from build123d import *

# Parameters (mm, degrees)
SKETCH1_R           = 1.077630735
BOSS_EXTRUDE1_DEPTH = 8.001
SKETCH4_R           = 2.032
CUT_EXTRUDE1_DEPTH  = 50.8
SKETCH5_R           = 3.048
CUT_EXTRUDE2_DEPTH  = 4.572
CUT_EXTRUDE4_DEPTH  = 34.909144773
FILLET2_R           = 5.08
FILLET3_R           = 1.6002
CHAMFER1_SIZE       = 0.508


with BuildPart() as part:
    # Sketch1 → Boss-Extrude1 (new body)
    with BuildSketch(Plane(origin=(0, 0, 0), x_dir=(1, 0, 0), z_dir=(0, 1, 0))):
        with BuildLine():
            Line((-0.609859659, 0), (0, 0))
            Line((0, 0), (4.662509606, 0))
            Line((4.662509606, 0), (4.662509606, -27.178))
            Line((4.662509606, -27.178), (8.472509606, -27.178))
            Line((8.472509606, -27.178), (8.472509606, 7.747))
            Line((8.472509606, 7.747), (4.535509606, 7.747))
            Line((4.535509606, 7.747), (-1.371859637, 1.839630756))
            ThreePointArc((-1.371859637, 1.839630756), (-0.197468217, 2.073231708), (0.467771075, 1.077630735))
            ThreePointArc((0.467771075, 1.077630735), (0.152140341, 0.315630735), (-0.609859659, 0))
        make_face()
        with Locations((-0.609859659, 1.077630735)):
            Circle(SKETCH1_R)
    boss_extrude1 = extrude(amount=BOSS_EXTRUDE1_DEPTH)

    # Mirror1: Boss-Extrude1 across plane
    add(boss_extrude1.mirror(Plane(origin=(8.472509606, 0, 0), x_dir=(0, 0, 1), z_dir=(1, 0, 0))))

    # Sketch4 → Cut-Extrude1 (cut)
    with BuildSketch(Plane(origin=(0, 0, -7.747), x_dir=(-1, 0, 0), z_dir=(0, 0, -1))):
        with Locations((-8.472509606, 4.0005)):
            Circle(SKETCH4_R)
    extrude(amount=-CUT_EXTRUDE1_DEPTH, mode=Mode.SUBTRACT)

    # Sketch5 → Cut-Extrude2 (cut)
    with BuildSketch(Plane(origin=(0, 0, -7.747), x_dir=(-1, 0, 0), z_dir=(0, 0, -1))):
        with Locations((-8.472509606, 4.0005)):
            Circle(SKETCH5_R)
    extrude(amount=-CUT_EXTRUDE2_DEPTH, mode=Mode.SUBTRACT)

    # Sketch7 → Cut-Extrude4 (cut, through all)
    with BuildSketch(Plane(origin=(0, 8.001, 0), x_dir=(1, 0, 0), z_dir=(0, 1, 0))):
        with BuildLine():
            ThreePointArc((9.272609606, -24.93293597), (8.166324592, -24.193739956), (7.906753471, -25.498692105))
            Line((7.906753471, -25.498692105), (8.472509606, -24.93293597))
            Line((8.472509606, -24.93293597), (9.038265742, -25.498692105))
            ThreePointArc((9.038265742, -25.498692105), (9.21170562, -25.239120984), (9.272609606, -24.93293597))
        make_face()
        with BuildLine():
            Line((8.472509606, -24.93293597), (7.906753471, -25.498692105))
            ThreePointArc((7.906753471, -25.498692105), (8.472509606, -25.73303597), (9.038265742, -25.498692105))
            Line((9.038265742, -25.498692105), (8.472509606, -24.93293597))
        make_face()
        with BuildLine():
            Line((7.906753471, -25.498692105), (6.227445576, -27.178))
            Line((6.227445576, -27.178), (10.717573636, -27.178))
            Line((10.717573636, -27.178), (9.038265742, -25.498692105))
            ThreePointArc((9.038265742, -25.498692105), (8.472509606, -25.73303597), (7.906753471, -25.498692105))
        make_face()
    extrude(amount=-CUT_EXTRUDE4_DEPTH, mode=Mode.SUBTRACT)

    # Fillet2
    # the kernel refuses this fillet: 5.08 mm, written as the material it takes off along each edge
    with BuildSketch(Plane(origin=(4.535509606, -5.260512242, -7.747), x_dir=(-0.7071067811865458, 0, 0.7071067811865495), z_dir=(0, 1, 0)), Plane(origin=(12.409509606, -5.260512242, -7.747), x_dir=(-1, 0, 0), z_dir=(0, 1, 0))) as fillet2_piece_1:
        with BuildLine():
            CenterArc((FILLET2_R * 0.414213562373, FILLET2_R), FILLET2_R, 225, 45)
            Line((-FILLET2_R * 0.292893218813, FILLET2_R * 0.292893218813), (0, 0))
            Line((0, 0), (FILLET2_R * 0.414213562373, 0))
        make_face()
    extrude(amount=18.522024484, mode=Mode.SUBTRACT)

    # Fillet3
    fillet3_edges = [part.edges().sort_by_distance(p)[0] for p in [
        (4.662509606, 4.0005, 0),
        (12.282509606, 4.0005, 0),
    ]]
    fillet(fillet3_edges, radius=FILLET3_R)

    # Chamfer1
    chamfer1_edges = [part.edges().sort_by_distance(p)[0] for p in [
        (15.718794239, 0, 0),
        (15.718794239, 8.001, 0),
        (12.282509606, 0, 14.3891),
        (12.282509606, 8.001, 14.3891),
        (4.662509606, 0, 14.3891),
        (4.662509606, 8.001, 14.3891),
        (-1.605460644, 0, -0.66523932),
        (1.226224973, 0, 0),
        (1.226224973, 8.001, 0),
        (12.751197335, 0, 0.468687729),
        (12.751197335, 8.001, 0.468687729),
        (4.193821877, 0, 0.468687729),
        (4.193821877, 8.001, 0.468687729),
        (0.837876209, 0, -4.049366602),
        (16.107143004, 0, -4.049366602),
        (18.550479857, 8.001, -0.66523932),
        (16.107143004, 8.001, -4.049366602),
        (18.550479857, 0, -0.66523932),
        (0.837876209, 8.001, -4.049366602),
        (-1.605460644, 8.001, -0.66523932),
        (8.472509606, 0, -7.747),
        (12.249336546, 0, -7.360308025),
        (4.695682667, 0, -7.360308025),
        (8.472509606, 8.001, -7.747),
        (12.249336546, 8.001, -7.360308025),
        (4.695682667, 8.001, -7.360308025),
    ]]
    chamfer(chamfer1_edges, length=CHAMFER1_SIZE)


solid = part.part
The model under review builds one solid part; all positions refer to its coordinate system, in mm. A direction names the side the tool comes from. Round coordinates to 2 decimals unless told otherwise and drop trailing zeros. Loops run counter-clockwise (first coordinate to the right, second up) from the corner with the lowest first, then second, coordinate; pieces in that order, holes last. Notation, with made-up numbers: (-23, -30.5) -> (-6, -30.5) arc R27 ccw to (-6, -14.5) -> close; hole circle Ø10 at (40.5, -22.75). An arc over 180 degrees is marked (long way). Answer as CSV lines item,"result".
1) Add section D-D on y = 4.75. Write out the cut boundary in (x, z) (1 decimal), plus the area to 3 significant figures.
Geometry results:
outline,"(-1.4, -1.8) -> (3, -6.3) arc R5.1 ccw to (5.5, -7.6) -> (5.5, -3.2) -> (6.6, -3.2) -> (6.6, 26.8) -> (6.2, 27.2) -> (4.7, 27.2) -> (4.7, 1.6) arc R1.6 cw to (3.1, 0) -> (-0.6, 0) arc R1.1 ccw to start; (10.4, -3.2) -> (11.4, -3.2) -> (11.4, -7.6) arc R5.1 ccw to (13.9, -6.3) -> (18.3, -1.8) arc R1.1 ccw to (17.6, 0) -> (13.9, 0) arc R1.6 cw to (12.3, 1.6) -> (12.3, 27.2) -> (10.7, 27.2) -> (10.4, 26.8) -> close"
area,"184 mm²"
2) Tool access review of faces 4 (the face through (1, 4, 0)), 5 (the face through (6.519, 4.946, 26.886)), 6 (the face through (16, 4, 0)): name each direction out of +Z, -Z, +X, -X, +Y, -Y from which nothing blocks a thin tool from reaching the whole face with its end or side.
Geometry results:
face 4,"+Z, -X, +Y, -Y"
face 5,"+Z, +Y, -Y"
face 6,"+Z, +X, +Y, -Y"
3) Add section B-B on z = 17. Write out the cut boundary in (x, y), plus the area to 3 significant figures.
Geometry results:
outline,"(4.66, 0.51) -> (5.17, 0) -> (11.77, 0) -> (12.28, 0.51) -> (12.28, 7.49) -> (11.77, 8) -> (5.17, 8) -> (4.66, 7.49) -> close; hole circle Ø4.06 at (8.47, 4)"
area,"47.5 mm²"
4) Add section C-C on x = 16.75. Write out the cut boundary in (y, z).
Geometry results:
outline,"(0, -2.69) -> (0.51, -3.41) -> (7.49, -3.41) -> (8, -2.69) -> (8, -0.51) -> (7.49, 0) -> (0.51, 0) -> (0, -0.51) -> close"
5) Add section A-A on y = 2.5. Write out the cut boundary in (x, z) (1 decimal).
Geometry results:
outline,"(-1.4, -1.8) -> (3, -6.3) arc R5.1 ccw to (5.8, -7.7) -> (5.8, -3.2) -> (7.1, -3.2) -> (7.1, 26.3) -> (6.2, 27.2) -> (4.7, 27.2) -> (4.7, 1.6) arc R1.6 cw to (3.1, 0) -> (-0.6, 0) arc R1.1 ccw to start; (9.8, -3.2) -> (11.1, -3.2) -> (11.1, -7.7) arc R5.1 ccw to (13.9, -6.3) -> (18.3, -1.8) arc R1.1 ccw to (17.6, 0) -> (13.9, 0) arc R1.6 cw to (12.3, 1.6) -> (12.3, 27.2) -> (10.7, 27.2) -> (9.8, 26.3) -> close"
6) To check wall thickness, follow line 1 along X through (y, z) = (7.5, 13); line 2 along Y through (x, z) = (9, -6); line 3 along Y through (x, z) = (7.5, 13.5). State the ranges of each line that lie inside material, in increasing order. Write a range as from..to.
Geometry results:
line 1,"x = 4.67..12.28"
line 2,"y = 0..1, 7..8"
line 3,"y = 0..2.22, 5.78..8"
7) Draft analysis for pull direction Y (two halves, no side actions). For faces 1 (the face through (-1.259, 7.863, -0.796)), 2 (the face through (12.1, 0.19, -7.08)), 3 (the face through (9, 1, -5)), state which applies: pulls with the +Y half, pulls with the -Y half, needs draft (parallel to the pull), parting line crosses it, or undercut.
Geometry results:
face 1,"pulls with the +Y half"
face 2,"pulls with the -Y half"
face 3,"undercut"
8) For P1, Ø1.8, axis at x = 8.47, z = 24.93, coming from the -Y side; P2, Ø4, axis at x = 0.5, y = 4.5, coming from the +Z side; P3, Ø2, axis at x = 3, y = 3.5, coming from the -Z side; P4, Ø1, axis at y = 2.5, z = 19, coming from the +X side, all flat-tipped, find the tip position at first contact; note any pin that passes through.
Geometry results:
P1,"stops at y = 0"
P2,"stops at z = 0"
P3,"stops at z = -7.01"
P4,"stops at x = 12.28"
